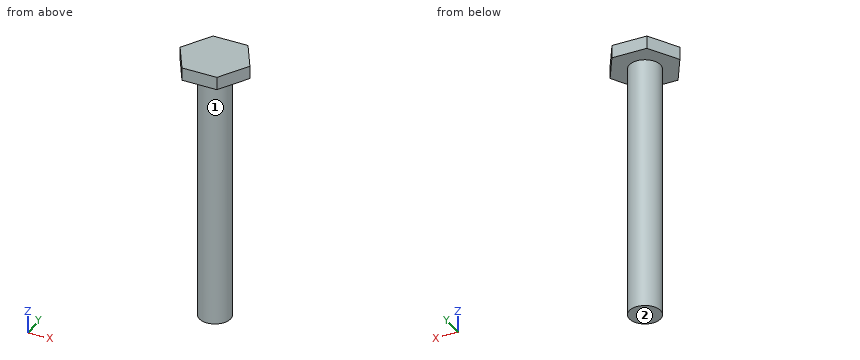
```python
from build123d import *

# Parameters (mm, degrees)
F0_W     = 2
F0_H     = 3.5
F0_W_2   = 4.25
F0_H_2   = 36
F0_H_3   = 34
F3_DEPTH = 73.5


with BuildPart() as f1:
    # F0 (on Front) → F1 (revolve)
    with BuildSketch(Plane.XZ):
        Polygon((-4.25, 35), (0, 35), (0, 38.5), (-7.5, 38.5), (-7.5, 35), align=None)
        with Locations((-8.5, 36.75)):
            Rectangle(F0_W, F0_H)
        with Locations((-2.125, 17)):
            Rectangle(F0_W_2, F0_H_2)
        with Locations((-2.125, -18)):
            Rectangle(F0_W_2, F0_H_3)
    revolve(axis=Axis((0, 0, 36.75), (0, 0, 1)))

    # F2 (on face) → F3 (intersect, through all)
    with BuildSketch(Plane.XY.offset(38.5)):
        Polygon((4.75, -8.227241), (9.5, 0), (4.75, 8.227241), (-4.75, 8.227241), (-9.5, 0), (-4.75, -8.227241), align=None)
    extrude(amount=-F3_DEPTH, mode=Mode.INTERSECT)


solid = f1.part
```
Input: part model. Units: mm. Frame: model coordinates. Face numbers are marked on the shaded views. A direction names the side the tool comes from. Round coordinates to 2 decimals unless told otherwise and drop trailing zeros. Loops run counter-clockwise (first coordinate to the right, second up) from the corner with the lowest first, then second, coordinate; pieces in that order, holes last. Notation, with made-up numbers: M 2,33.5 L 48,33.5 A26 cw 48,62.5 Z; hole C 28,64 d8. An arc over 180 degrees is marked long. Answer in a Markdown table with one row per item. Add a question column.
1. Section C-C (z = -15.5). Output: boundary loops of the cut face in (x, y), and give its area (3 significant figures).
2. Set-up query: the marked faces 1 and 2. Return all of +Z, -Z, +X, -X, +Y, -Y with unobstructed straight access to the full face (end or side cutting, diameter ignored); none if empty.
3. Section D-D (y = -6.5). Output: boundary loops of the cut face in (x, z), and give its area (3 significant figures).
4. Contact query for flat-ended pins moving along their axis: pin 1 (5 mm diameter, centred on y = -4.5, z = -16.5, fed in from -X); pin 2 (6 mm diameter, centred on y = 5, z = -2.5, fed in from +X); pin 3 (8 mm diameter, centred on x = 3.5, z = -16, fed in from +Y). Output: stop coordinate, or through.
5. Section B-B (y = -1.25). Output: boundary loops of the cut face in (x, z).
6. Ray query, probe 1 along Z at (x, y) = (5, 0); probe 2 along X at (y, z) = (-0.25, 9); probe 3 along Y at (x, z) = (0.75, 28.5). Return the intervals inside material, ascending.
7. Section A-A (x = 0). Output: boundary loops of the cut face in (y, z).
Values follow:
| question | item | result |
|---|---|---|
| 1 | outline | C 0,0 d8.5 |
| 1 | area | 56.7 mm^2 |
| 2 | face 1 | -Z |
| 2 | face 2 | -Z, +X, -X, +Y, -Y |
| 3 | outline | M -5.75,35 L 5.75,35 L 5.75,38.5 L -5.75,38.5 Z |
| 3 | area | 40.2 mm^2 |
| 4 | pin 1 | x = -3.75 |
| 4 | pin 2 | x = 3.75 |
| 4 | pin 3 | y = 4.25 |
| 5 | outline | M -8.78,35 L -4.06,35 L -4.06,-35 L 4.06,-35 L 4.06,35 L 8.78,35 L 8.78,38.5 L -8.78,38.5 Z |
| 6 | probe 1 | 35 to 38.5 |
| 6 | probe 2 | -4.24 to 4.24 |
| 6 | probe 3 | -4.18 to 4.18 |
| 7 | outline | M -8.23,35 L -4.25,35 L -4.25,-35 L 4.25,-35 L 4.25,35 L 8.23,35 L 8.23,38.5 L -8.23,38.5 Z |
